from build123d import *

# Parameters (mm, degrees)
F0_W     = 15.0114
F0_H     = 17.4625
F0_W_2   = 7.2136
F0_H_2   = 10.287
F2_R     = 1.5875
F3_SIZE  = 0.79375
F4_SIZE2 = 6.35
F4_SIZE  = 1.5748


with BuildPart() as f1:
    # F0 (on Right) → F1 (revolve)
    with BuildSketch(Plane.YZ):
        with Locations((14.7193, 16.66875)):
            Rectangle(F0_W, F0_H)
        with Locations((3.6068, 16.66875)):
            Rectangle(F0_W_2, F0_H)
        with Locations((3.6068, 30.5435)):
            Rectangle(F0_W_2, F0_H_2)
    revolve(axis=Axis((0, 9.448286066, 0), (0, 1, 0)))

    # F2
    f2_edges = [f1.edges().sort_by_distance(p)[0] for p in [
        (0, 7.2136, -25.4),
    ]]
    fillet(f2_edges, radius=F2_R)

    # F3
    f3_edges = [f1.edges().sort_by_distance(p)[0] for p in [
        (0, 22.225, -7.9375),
        (0, 22.225, -25.4),
    ]]
    chamfer(f3_edges, length=F3_SIZE)

    # F4
    f4_edges = [f1.edges().sort_by_distance(p)[0] for p in [
        (0, 0, -35.687),
        (0, 7.2136, -35.687),
    ]]
    f4_side = f1.faces().sort_by_distance((0, 3.6068, -35.687))[0]
    chamfer(f4_edges, length=F4_SIZE, length2=F4_SIZE2, reference=f4_side)


solid = f1.part
Can you work these out from the model? Positions are in its coordinate system, mm. A direction names the side the tool comes from. Give positions to 0.01 mm unless a question says otherwise; leave off trailing zeros. Order: outer loops, then holes, each group sorted by start corner. A loop starts at its lowest first (then second) coordinate and runs counter-clockwise, first axis right, second up. Notation, with made-up numbers: M -0.5,13.5 L 47.5,13.5 A16 cw 47.5,42.5 Z; hole C -32.75,9 d4. An arc over 180 degrees is marked long. Use one line per item in the form item = value.
Item 1: Will these pins go through, and if not, where does the flat tip stop? pin 1 Ø6 at (x, y) = (9.5, 11) entering from -Z; pin 2 Ø3 at (x, z) = (19.5, -26.5) entering from -Y; pin 3 Ø3 at (y, z) = (10, -1) entering from +X.
Values follow:
pin_1 = -24.55
pin_2 = 0.51
pin_3 = 25.41
Item 2: If we section it at C-C, the plane y = 12.5: Write out the boundary of the cut face in (x, z) (1 decimal), and give its area (3 significant figures).
Values follow:
outline = C 0,0 d50.8; hole C 0,0 d15.9
area = 1,830 mm^2
Item 3: If we section it at D-D, the plane y = 4.25: Write out the boundary of the cut face in (x, z) (1 decimal).
Values follow:
outline = C 0,0 d71.4; hole C 0,0 d15.9
Item 4: If I drill on line 1 along X through (y, z) = (14.75, 0); line 2 along X through (y, z) = (5, 0); line 3 along Z through (x, y) = (-3, 15.5), over which ranges is the centre line in solid material (lowest first)? Write a range as [from, to].
Values follow:
line_1 = [-25.4, -7.94], [7.94, 25.4]
line_2 = [-35.69, -7.94], [7.94, 35.69]
line_3 = [-25.22, -7.35], [7.35, 25.22]
Item 5: If we section it at B-B, the plane x = 0: Write out the boundary of the cut face in (y, z) (1 decimal).
Values follow:
outline = M 0,-29.3 L 1.6,-35.7 L 5.6,-35.7 L 7.2,-29.3 L 7.2,-27 A1.6 cw 8.8,-25.4 L 21.4,-25.4 L 22.2,-24.6 L 22.2,-8.7 L 21.4,-7.9 L 0,-7.9 Z; M 0,7.9 L 21.4,7.9 L 22.2,8.7 L 22.2,24.6 L 21.4,25.4 L 8.8,25.4 A1.6 cw 7.2,27 L 7.2,29.3 L 5.6,35.7 L 1.6,35.7 L 0,29.3 Z
Item 6: For faces 1 (the conical face through (-28.94, 0.076, -6.427)), 2 (the flat face through (-24, 7.214, -13)), which set-ups out of +Z, -Z, +X, -X, +Y, -Y let a thin tool reach every point of the face, with its end or its side?
Values follow:
face_1 = -Y
face_2 = +Y
Item 7: Thinking about a two-plate mould opening in X: for faces 3 (the cylindrical face through (-7.75, 10.87, -1.72)), 4 (the flat face through (-6, 0, 6)), 5 (the cylindrical face through (-24.796, 15.028, -5.506)), which applies, pulls with the +X half, pulls with the -X half, needs draft (parallel to the pull), parting line crosses it, or undercut?
Values follow:
face_3 = undercut
face_4 = needs draft
face_5 = parting line crosses it
Item 8: If we section it at A-A, the plane z = 0: Write out the boundary of the cut face in (x, y) (1 decimal).
Values follow:
outline = M -35.7,1.6 L -29.3,0 L -7.9,0 L -7.9,21.4 L -8.7,22.2 L -24.6,22.2 L -25.4,21.4 L -25.4,8.8 A1.6 cw -27,7.2 L -29.3,7.2 L -35.7,5.6 Z; M 7.9,0 L 29.3,0 L 35.7,1.6 L 35.7,5.6 L 29.3,7.2 L 27,7.2 A1.6 cw 25.4,8.8 L 25.4,21.4 L 24.6,22.2 L 8.7,22.2 L 7.9,21.4 Z
